For this review, take the finished solid that the model builds, in its own axes (mm). Face numbers are marked on the shaded views. A direction names the side the tool comes from. Coordinates: 2 decimals unless noted, no trailing zeros. Write each loop counter-clockwise with the first axis right and the second up, starting at its lowest first coordinate (ties: lowest second). Pieces come first, ordered by that corner, then holes.
1) Mouldability with a two-part tool opening along X and no side actions: class the marked faces 5, 6, 7 and 8 as pulls with the +X half, pulls with the -X half, needs draft (parallel to the pull), parting line crosses it, or undercut.
2) Insertion check: P1, Ø2, axis at y = 1, z = 5, coming from the -X side; P2, Ø1, axis at y = 5, z = -0.5, coming from the -X side (3 decimals). Each pin has a flat end and moves straight along its axis. Give the tip position at first contact, or say it passes through.
3) We need section C-C on x = -4.75. Write out the cut boundary in (y, z), then the cut area to 3 significant figures.
4) We need section B-B on z = 5.5. Write out the cut boundary in (x, y).
5) To check wall thickness, follow line 1 along Y through (x, z) = (-1, -0.75); line 2 along Y through (x, z) = (-1, 4.75); line 3 along Z through (x, y) = (0, 5.5) (3 decimals). State the ranges of each line that lie inside material, in increasing order.
6) For the marked faces 1, 2, 3 and 4, list the 3-axis set-ups (+Z, -Z, +X, -X, +Y, -Y) from which the entire face can be reached by the end or side of a thin tool; tool diameter is ignored.
7) We need section A-A on y = 4.5. Write out the cut boundary in (x, z) (3 decimals), then the cut area to 3 significant figures.
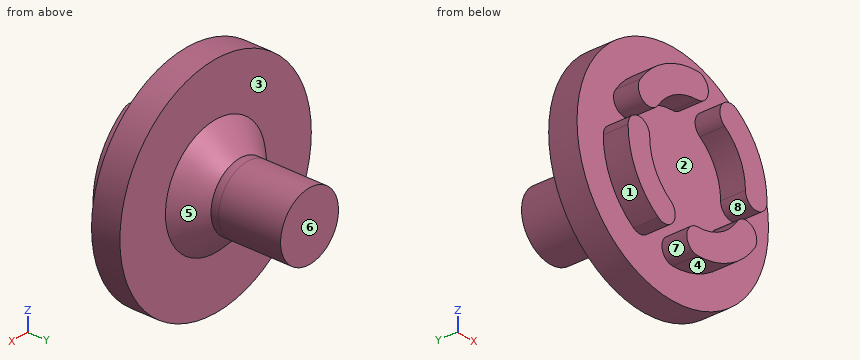
from build123d import *

# Parameters (mm, degrees)
ESQUISSE1_R        = 6.2
BOSS_EXTRU_1_DEPTH = 1.6
ESQUISSE2_R        = 1.875
BOSS_EXTRU_3_DEPTH = 5.3
ESQUISSE3_R        = 3.25
BOSS_EXTRU_5_DEPTH = 1.8
CHANFREIN2_SIZE    = 1.8
BOSS_EXTRU_6_DEPTH = 1.4


with BuildPart() as part:
    # Esquisse1 → Boss.-Extru.1 (new body)
    with BuildSketch(Plane(origin=(0, 0, 0), x_dir=(1, 0, 0), z_dir=(0, 1, 0))):
        with Locations(Location((0, 0, 0), (0, 0, 270))):
            Circle(ESQUISSE1_R)
    extrude(amount=BOSS_EXTRU_1_DEPTH)

    # Esquisse2 → Boss.-Extru.3 (add)
    with BuildSketch(Plane(origin=(0, 1.6, 0), x_dir=(1, 0, 0), z_dir=(0, 1, 0))):
        with Locations(Location((0, 0, 0), (0, 0, 270))):
            Circle(ESQUISSE2_R)
    extrude(amount=BOSS_EXTRU_3_DEPTH)

    # Esquisse3 → Boss.-Extru.5 (add)
    with BuildSketch(Plane(origin=(0, 1.6, 0), x_dir=(1, 0, 0), z_dir=(0, 1, 0))):
        with Locations(Location((0, 0, 0), (0, 0, 270))):
            Circle(ESQUISSE3_R)
    extrude(amount=BOSS_EXTRU_5_DEPTH)

    # Chanfrein2
    # the kernel refuses this chamfer: 1.8 mm, written as the material it takes off along each edge
    with BuildSketch(Plane(origin=(0, 3.4, 0), x_dir=(0, 0, 1), z_dir=(-1, 0, 0))) as chanfrein2_piece_1_section:
        Polygon((3.25, -CHANFREIN2_SIZE), (3.25 - CHANFREIN2_SIZE, 0), (3.25, 0), align=None)
    chanfrein2_piece_1 = revolve(axis=Axis((0, 3.4, 0), (0, 1, 0)), mode=Mode.PRIVATE)
    chanfrein2_piece_1 = split(chanfrein2_piece_1, bisect_by=Plane(origin=(0, 1.6, -2.584069467), z_dir=(0, 1, 0)), keep=Keep.TOP, mode=Mode.PRIVATE)
    chanfrein2_piece_1 = chanfrein2_piece_1 - Plane(origin=(0, 2.309069467, 0), x_dir=(0, 0, 1), z_dir=(0, -1, 0)) * Cylinder(1.875, 13, mode=Mode.PRIVATE)
    add(chanfrein2_piece_1, mode=Mode.SUBTRACT)

    # Esquisse4 → Boss.-Extru.6 (add)
    with BuildSketch(Plane.XZ):
        with BuildLine():
            ThreePointArc((0, -4.5), (2.098884425, -3.980538176), (3.71319537, -2.542081853))
            ThreePointArc((3.71319537, -2.542081853), (3.531022156, -1.569038729), (2.557979032, -1.751211943))
            ThreePointArc((2.557979032, -1.751211943), (1.44589816, -2.742148521), (0, -3.1))
            ThreePointArc((0, -3.1), (-0.7, -3.8), (0, -4.5))
        make_face()
        with BuildLine():
            ThreePointArc((3.1, 0), (3.8, -0.7), (4.5, 0))
            ThreePointArc((4.5, 0), (3.980538176, 2.098884425), (2.542081853, 3.71319537))
            ThreePointArc((2.542081853, 3.71319537), (1.569038729, 3.531022156), (1.751211943, 2.557979032))
            ThreePointArc((1.751211943, 2.557979032), (2.742148521, 1.44589816), (3.1, 0))
        make_face()
        with BuildLine():
            ThreePointArc((-4.5, 0), (-3.980538176, -2.098884425), (-2.542081853, -3.71319537))
            ThreePointArc((-2.542081853, -3.71319537), (-1.569038729, -3.531022156), (-1.751211943, -2.557979032))
            ThreePointArc((-1.751211943, -2.557979032), (-2.742148521, -1.44589816), (-3.1, 0))
            ThreePointArc((-3.1, 0), (-3.8, 0.7), (-4.5, 0))
        make_face()
        with BuildLine():
            ThreePointArc((0, 3.1), (0.7, 3.8), (0, 4.5))
            ThreePointArc((0, 4.5), (-2.098884425, 3.980538176), (-3.71319537, 2.542081853))
            ThreePointArc((-3.71319537, 2.542081853), (-3.531022156, 1.569038729), (-2.557979032, 1.751211943))
            ThreePointArc((-2.557979032, 1.751211943), (-1.44589816, 2.742148521), (0, 3.1))
        make_face()
    extrude(amount=BOSS_EXTRU_6_DEPTH)


solid = part.part
Result:
1. face 5: parting line crosses it
1. face 6: needs draft
1. face 7: undercut
1. face 8: undercut
2. P1: stops at x = -4.74
2. P2: stops at x = -1.875
3. outline: (0, -3.98) - (1.6, -3.98) - (1.6, 3.98) - (0, 3.98) - close
3. area: 12.8 mm2
4. outline: (-2.86, 0) - (2.86, 0) - (2.86, 1.6) - (-2.86, 1.6) - close
5. line 1: y = 0 to 6.9
5. line 2: y = 0 to 1.6
5. line 3: z = -1.875 to 1.875
6. face 1: -Z, -X, -Y
6. face 2: -Y
6. face 3: +Y
6. face 4: -Z, +X, -Y
7. outline: circle Ø3.75 at (0, 0)
7. area: 11.0 mm2
